```python
from build123d import *

# Parameters (mm, degrees)
F0_R     = 25.4
F0_W     = 3.81
F0_H     = 19.05
F0_W_2   = 60.325
F0_H_2   = 153.5942826
F1_DEPTH = 3.429


# Not quite as in the source:
# - ends of sketch curves that miss each other by under 0.0002 mm in the source are joined


with BuildPart() as f1:
    # F0 (on Front) → F1 (new body)
    with BuildSketch(Plane.XZ):
        with BuildLine():
            Line((68.2613062, -217.1147804), (68.2613062, -246.3247804))
            Line((68.2613062, -246.3247804), (143.8263062, -246.3247804))
            Line((143.8263062, -246.3247804), (143.8263062, -243.1497804))
            Line((143.8263062, -243.1497804), (162.8763062, -243.1497804))
            Line((162.8763062, -243.1497804), (162.8763062, -246.3247804))
            Line((162.8763062, -246.3247804), (371.7913062, -246.3247804))
            Line((371.7913062, -246.3247804), (371.7913062, -112.9747804))
            Line((371.7913062, -112.9747804), (406.7163062, -112.9747804))
            Line((406.7163062, -112.9747804), (406.7163062, -246.3247804))
            Line((406.7163062, -246.3247804), (452.4363062, -246.3247804))
            Line((452.4363062, -246.3247804), (452.4363062, -243.1497804))
            Line((452.4363062, -243.1497804), (471.4863062, -243.1497804))
            Line((471.4863062, -243.1497804), (471.4863062, -246.3247804))
            Line((471.4863062, -246.3247804), (761.0463062, -246.3247804))
            Line((761.0463062, -246.3247804), (761.0463062, -243.1497804))
            Line((761.0463062, -243.1497804), (780.0963062, -243.1497804))
            Line((780.0963062, -243.1497804), (780.0963062, -246.3247804))
            Line((780.0963062, -246.3247804), (855.6613062, -246.3247804))
            Line((855.6613062, -246.3247804), (855.6613062, -217.1147804))
            Line((855.6613062, -217.1147804), (858.8363062, -217.1147804))
            Line((858.8363062, -217.1147804), (858.8363062, -199.3347804))
            Line((858.8363062, -199.3347804), (855.6613062, -199.3347804))
            Line((855.6613062, -199.3347804), (855.6613062, -170.1247804))
            Line((855.6613062, -170.1247804), (688.2210772, -153.9405354))
            ThreePointArc((688.2210772, -153.9405354), (602.6698633523, -117.0648991424), (554.5656172379, -37.2851738969))
            ThreePointArc((554.5656172379, -37.2851738969), (545.6072798598, -23.2063701747), (529.846032, -17.7247804))
            Line((529.846032, -17.7247804), (394.0766058, -17.7247804))
            ThreePointArc((394.0766058, -17.7247804), (378.3153579402, -23.2063701747), (369.3569994588, -37.2851689116))
            ThreePointArc((369.3569994588, -37.2851689116), (321.2527512475, -117.0648972224), (235.7015357309, -153.9405408928))
            Line((235.7015357309, -153.9405408928), (68.2613062, -170.1247804))
            Line((68.2613062, -170.1247804), (68.2613062, -199.3347804))
            Line((68.2613062, -199.3347804), (65.0863062, -199.3347804))
            Line((65.0863062, -199.3347804), (65.0863062, -217.1147804))
            Line((65.0863062, -217.1147804), (68.2613062, -217.1147804))
        make_face()
        with Locations((106.5103026, -207.9172118)):
            Circle(F0_R, mode=Mode.SUBTRACT)
        with Locations((169.8620428, -207.9172118)):
            Circle(F0_R, mode=Mode.SUBTRACT)
        with Locations((199.9603062, -206.9547804)):
            Rectangle(F0_W, F0_H, mode=Mode.SUBTRACT)
        with Locations((233.3611284, -207.9172118)):
            Circle(F0_R, mode=Mode.SUBTRACT)
        with Locations((296.9567594, -207.9172118)):
            Circle(F0_R, mode=Mode.SUBTRACT)
        with Locations((349.1853062, -182.1897804)):
            Rectangle(F0_W, F0_H, mode=Mode.SUBTRACT)
        with Locations((626.9658784, -207.9172118)):
            Circle(F0_R, mode=Mode.SUBTRACT)
        with Locations((690.5615094, -207.9172118)):
            Circle(F0_R, mode=Mode.SUBTRACT)
        with Locations((723.9623062, -206.9547804)):
            Rectangle(F0_W, F0_H, mode=Mode.SUBTRACT)
        with Locations((754.0605696, -207.9172118)):
            Circle(F0_R, mode=Mode.SUBTRACT)
        with Locations((817.4123352, -207.9172118)):
            Circle(F0_R, mode=Mode.SUBTRACT)
        with Locations((574.7373062, -182.1897804)):
            Rectangle(F0_W, F0_H, mode=Mode.SUBTRACT)
        with Locations((461.9613062, -100.8605933)):
            Rectangle(F0_W_2, F0_H_2, mode=Mode.SUBTRACT)
    extrude(amount=F1_DEPTH)


solid = f1.part
```
Can you work these out from the model? Positions are in its coordinate system, mm. Give positions to 0.01 mm unless a question says otherwise; leave off trailing zeros. Order: outer loops, then holes, each group sorted by start corner. A loop starts at its lowest first (then second) coordinate and runs counter-clockwise, first axis right, second up. Notation, with made-up numbers: M 2,-32 L 31,-32 A13 cw 31,-11 Z; hole C 79.5,87.5 d1. An arc over 180 degrees is marked long. Write item = value, one per line. Start each with the question number.
Q1. We'd pull the mould along X, two halves only. Please class faces 1 (the cylindrical face through (151.14, -1.69, -190.75)), 2 (the cylindrical face through (603.67, -1.69, -117.93)), 3 (the cylindrical face through (214.64, -1.69, -190.75)), 4 (the flat face through (456, 0, -181)): pulls with the +X half, pulls with the -X half, needs draft (parallel to the pull), parting line crosses it, or undercut.
Q2. I need wall thicknesses on probe 1 along X at (y, z) = (-3.3, -178.5); probe 2 along Z at (x, y) = (457, -2.7); probe 3 along Z at (x, y) = (451.5, -1.2). Which ranges of each line are inside material? Lowest first, please. Write a range as [from, to].
Q3. Suppose I cut it at C-C (z = -130). Write out the boundary of the cut face in (x, y), plus the area to 3 significant figures.
Q4. Will these pins go through, and if not, where does the flat tip stop? pin 1 Ø1.7 at (y, z) = (-2, -186) entering from +X; pin 2 Ø1.6 at (y, z) = (-2, -244.5) entering from -X; pin 3 Ø1.7 at (x, y) = (382, -1) entering from -Z.
Q5. Suppose I cut it at B-B (x = 173). Write out the boundary of the cut face in (y, z), plus the area to 3 significant figures.
Q6. Suppose I cut it at A-A (z = -62). Write out the boundary of the cut face in (x, y), plus the area to 3 significant figures.
Q7. Suppose I cut it at D-D (y = -2.75). Count the separate pieces of the cut face and the enclosed holes in it, plus the area to 3 significant figures.
Check result:
q1.face_1 = undercut
q1.face_2 = pulls with the +X half
q1.face_3 = undercut
q1.face_4 = needs draft
q2.probe_1 = [68.26, 347.28], [351.09, 371.79], [406.72, 572.83], [576.64, 855.66]
q2.probe_2 = [-243.15, -177.66], [-24.06, -17.72]
q2.probe_3 = [-246.32, -177.66], [-24.06, -17.72]
q3.outline = M 304.14,-3.43 L 371.79,-3.43 L 371.79,0 L 304.14,0 Z; M 406.72,-3.43 L 431.8,-3.43 L 431.8,0 L 406.72,0 Z; M 492.12,-3.43 L 619.79,-3.43 L 619.79,0 L 492.12,0 Z
q3.area = 756 mm2
q4.pin_1 = 855.66
q4.pin_2 = 68.26
q4.pin_3 = -112.97
q5.outline = M -3.43,-246.32 L 0,-246.32 L 0,-233.12 L -3.43,-233.12 Z; M -3.43,-182.71 L 0,-182.71 L 0,-160 L -3.43,-160 Z
q5.area = 123 mm2
q6.outline = M 361.24,-3.43 L 431.8,-3.43 L 431.8,0 L 361.24,0 Z; M 492.12,-3.43 L 562.69,-3.43 L 562.69,0 L 492.12,0 Z
q6.area = 484 mm2
q7.separate_pieces = 1
q7.enclosed_holes = 13
q7.area = 73,200 mm2
